Verification items for the finished model (mm, model axes). A direction names the side the tool comes from. Give positions to 0.01 mm unless a question says otherwise; leave off trailing zeros. Write each loop counter-clockwise with the first axis right and the second up, starting at its lowest first coordinate (ties: lowest second). Pieces come first, ordered by that corner, then holes. Notation, with made-up numbers: (63.25, 25) - (87.25, 25) arc R30 cw to (87.25, 58) - close; hole circle Ø11 at (70.5, -13). An arc over 180 degrees is marked (long way). Answer as a JSON object with one key per item and string values. Group by question number.
Item 1: Sectioned sample at B-B, the plane z = 43. Record the boundary of the cut face in (x, y).
Item 2: Sectioned sample at A-A, the plane z = 60. Record the boundary of the cut face in (x, y), and give its area (3 significant figures).
Item 3: Tool access check on faces 4 (the face through (9.1, -9.1, 66.04)), 5 (the face through (10.368, -4.299, 57.826)). Record the directions out of +Z, -Z, +X, -X, +Y, -Y that give a thin tool (end or side, any length) a straight path to the whole face; none if there is none.
Item 4: Go/stop test with flat-tipped pins: pin 1 (3 mm diameter, centred on x = -1, z = 39, fed in from +Y); pin 2 (4 mm diameter, centred on x = -24.5, y = 14.5, fed in from -Z); pin 3 (4 mm diameter, centred on x = -12.5, z = 44, fed in from +Y); pin 4 (10 mm diameter, centred on y = -4.5, z = 52.5, fed in from -X). Record where each tip stops, or that it passes through.
Item 5: Scan lines: line 1 along Y through (x, z) = (0, 63); line 2 along Z through (x, y) = (2, -1.5); line 3 along Z through (x, y) = (-16.5, -0.5). Record each from-to range of solid material in increasing order. Write a range as [from, to].
Item 6: Draft check along Z on faces 1 (the face through (-5.17, -10.15, 67.31)), 2 (the face through (0, 0, 0)), 3 (the face through (0, 0, 2.54)). Enter one of: +Z half, -Z half, draft (parallel to the pull), parting line (faces both ways), or undercut.
```python
from build123d import *

# Parameters (mm, degrees)
F0_R      = 38.1
F2_R      = 12.7
F4_T      = -2.54
F5_R      = 12.7
F6_DEPTH  = 15.24
F7_R      = 10.5636642446
F8_DEPTH  = 53.34
F9_R      = 5.08
F10_SIZE  = 5.08
F11_R     = 13.7839746561
F12_DEPTH = 1.27
F13_R     = 11.2237856043
F14_DEPTH = 101.6
F16_R     = 11.2237856043
F17_DEPTH = 2.54


with BuildPart() as f3:
    # F0 (on Top) → F3 section 0
    with BuildSketch(Plane.XY):
        Circle(F0_R)
    # F2 (on offset) → F3 section 1
    with BuildSketch(Plane.XY.offset(50.8)):
        Circle(F2_R)
    loft()

    # F4
    f4_openings = [f3.faces().sort_by_distance(p)[0] for p in [
        (0, 0, 50.8),
    ]]
    offset(amount=F4_T, openings=f4_openings, kind=Kind.INTERSECTION)

    # F5 (on offset) → F6 (join)
    with BuildSketch(Plane.XY.offset(50.8)):
        Circle(F5_R)
    extrude(amount=F6_DEPTH)

    # F7 (on face) → F8 (cut)
    with BuildSketch(Plane.XY.offset(66.04)):
        Circle(F7_R)
    extrude(amount=-F8_DEPTH, mode=Mode.SUBTRACT)

    # F9
    f9_edges = [f3.edges().sort_by_distance(p)[0] for p in [
        (-38.1, 0, 0),
    ]]
    fillet(f9_edges, radius=F9_R)

    # F10
    f10_edges = [f3.edges().sort_by_distance(p)[0] for p in [
        (-12.7, 0, 50.8),
    ]]
    chamfer(f10_edges, length=F10_SIZE)

    # F11 (on face) → F12 (join)
    with BuildSketch(Plane.XY.offset(66.04)):
        Circle(F11_R)
    extrude(amount=F12_DEPTH)

    # F13 (on face) → F14 (cut)
    with BuildSketch(Plane.XY.offset(67.31)):
        Circle(F13_R)
    extrude(amount=-F14_DEPTH, mode=Mode.SUBTRACT)

    # F16 (on offset) → F17 (join)
    with BuildSketch(Plane.XY):
        Circle(F16_R)
    extrude(amount=F17_DEPTH)


solid = f3.part
```
Geometry check:
{
 "1": {"outline": "circle Ø33.2 at (0, 0); hole circle Ø27.52 at (0, 0)"},
 "2": {"outline": "circle Ø25.4 at (0, 0); hole circle Ø22.45 at (0, 0)", "area": "111 mm^2"},
 "3": {"face 4": "none", "face 5": "+Z"},
 "4": {"pin 1": "y = 19.33", "pin 2": "z = 0", "pin 3": "y = 12.65", "pin 4": "x = -14.38"},
 "5": {"line 1": "[-12.7, -11.22], [11.22, 12.7]", "line 2": "[0, 2.54]", "line 3": "[0, 2.54], [37.51, 43.18]"},
 "6": {"face 1": "+Z half", "face 2": "-Z half", "face 3": "undercut"}
}
